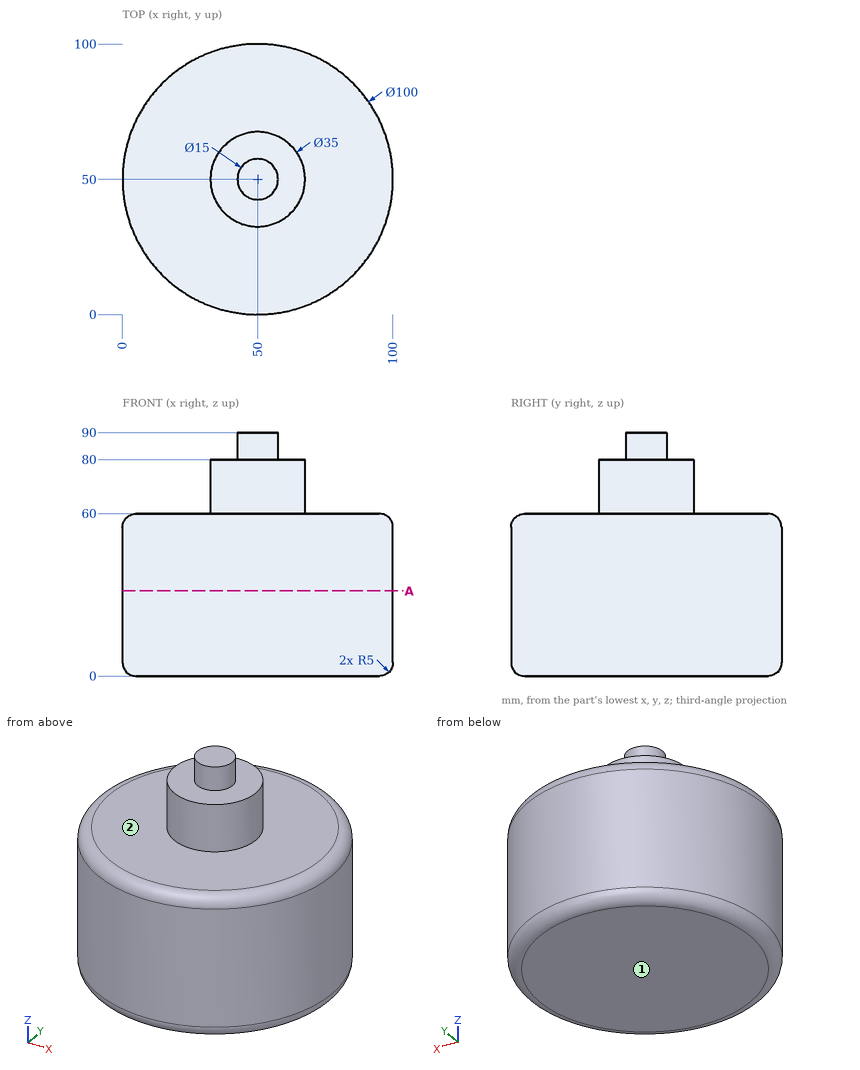
For this review, use the dimensioned drawing (mm, ordinates from the lowest corner) and the shaded views. A direction names the side the tool comes from. Round coordinates to 2 decimals unless told otherwise and drop trailing zeros. Loops run counter-clockwise (first coordinate to the right, second up) from the corner with the lowest first, then second, coordinate; pieces in that order, holes last. Notation, with made-up numbers: M -6,64 L -2,64 A27 ccw -2,92 Z; hole C -18,65 d2. An arc over 180 degrees is marked long. Answer as a JSON object with one key per item and string values.
(1) Clearance check with flat-ended pins moving along their axes: P1, Ø5, axis at x = 59, y = 50.5, coming from the +Z side; P2, Ø3, axis at y = 75.5, z = 24, coming from the +X side; P3, Ø6, axis at x = 17.5, z = 32.5, coming from the -Y side; P4, Ø6, axis at x = 13, z = 18.5, coming from the -Y side. State where each tip first meets the part, or that it passes through.
Resolved:
{"P1": "z = 90", "P2": "x = 93.86", "P3": "y = 9.63", "P4": "y = 13.34"}
(2) To check wall thickness, follow line 1 along X through (y, z) = (50.5, 27.5); line 2 along Y through (x, z) = (50.5, 73); line 3 along Z through (x, y) = (67, 70.5). State the ranges of each line that lie inside material, in increasing order.
Resolved:
{"line 1": "0 to 100", "line 2": "32.51 to 67.49", "line 3": "0 to 60"}
(3) Take a section at A-A on z = 31.5. Give the boundary of the cut face in (x, y), and give its area (3 significant figures).
Resolved:
{"outline": "C 50,50 d100", "area": "7,850 mm²"}
(4) Tool access review of the marked faces 1 and 2: name each direction out of +Z, -Z, +X, -X, +Y, -Y from which nothing blocks a thin tool from reaching the whole face with its end or side.
Resolved:
{"face 1": "-Z, +X, -X, +Y, -Y", "face 2": "+Z"}
